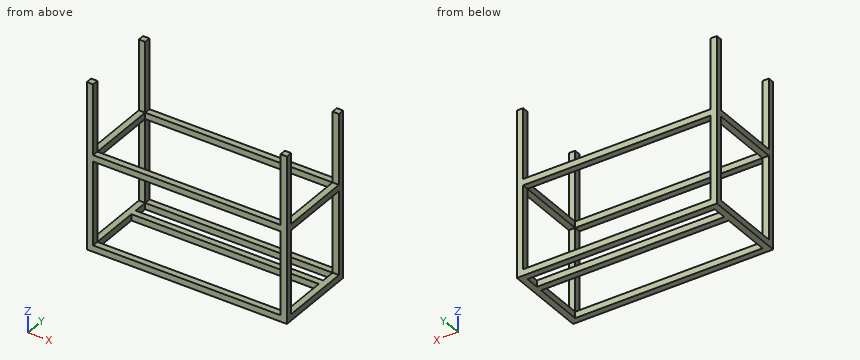
```python
from build123d import *

# Parameters (mm, degrees)
CROQUIS1_W              = 1200
CROQUIS1_H              = 500
CROQUIS1_W_2            = 1123.8
CROQUIS1_H_2            = 423.8
SALIENTE_EXTRUIR1_DEPTH = 38.1
CROQUIS2_W              = 38.1
CROQUIS2_H              = 38.1
SALIENTE_EXTRUIR2_DEPTH = 960
CROQUIS3_W              = 1123.8
CROQUIS3_H              = 38.1
SALIENTE_EXTRUIR4_DEPTH = 38.1
CROQUIS4_W              = 1123.8
CROQUIS4_H              = 38.1
SALIENTE_EXTRUIR5_DEPTH = 38.1
CROQUIS5_W              = 1123.8
CROQUIS5_H              = 38.1
SALIENTE_EXTRUIR6_DEPTH = 38.1
CROQUIS6_W              = 38.1
CROQUIS6_H              = 423.8
SALIENTE_EXTRUIR7_DEPTH = 38.1
CROQUIS7_W              = 38.1
CROQUIS7_H              = 423.8
SALIENTE_EXTRUIR8_DEPTH = 38.1


with BuildPart() as part:
    # Croquis1 → Saliente-Extruir1 (new body)
    with BuildSketch(Plane.XY):
        Rectangle(CROQUIS1_W, CROQUIS1_H)
        Rectangle(CROQUIS1_W_2, CROQUIS1_H_2, mode=Mode.SUBTRACT)
    extrude(amount=SALIENTE_EXTRUIR1_DEPTH)

    # Croquis2 → Saliente-Extruir2 (add)
    with BuildSketch(Plane.XY.offset(38.1)):
        with Locations((-580.95, 230.95)):
            Rectangle(CROQUIS2_W, CROQUIS2_H)
        with Locations((-580.95, -230.95)):
            Rectangle(CROQUIS2_W, CROQUIS2_H)
        with Locations((580.95, 230.95)):
            Rectangle(CROQUIS2_W, CROQUIS2_H)
        with Locations((580.95, -230.95)):
            Rectangle(CROQUIS2_W, CROQUIS2_H)
    extrude(amount=SALIENTE_EXTRUIR2_DEPTH)

    # Croquis3 → Saliente-Extruir4 (add)
    with BuildSketch(Plane(origin=(0, 0, 0), x_dir=(-1, 0, 0), z_dir=(0, 0, -1))):
        with Locations((0, 109.05)):
            Rectangle(CROQUIS3_W, CROQUIS3_H)
    extrude(amount=-SALIENTE_EXTRUIR4_DEPTH)

    # Croquis4 → Saliente-Extruir5 (add)
    with BuildSketch(Plane.XZ.offset(250)):
        with Locations((0, 557.15)):
            Rectangle(CROQUIS4_W, CROQUIS4_H)
    extrude(amount=-SALIENTE_EXTRUIR5_DEPTH)

    # Croquis5 → Saliente-Extruir6 (add)
    with BuildSketch(Plane(origin=(0, 250, 0), x_dir=(1, 0, 0), z_dir=(0, 1, 0))):
        with Locations((0, -557.15)):
            Rectangle(CROQUIS5_W, CROQUIS5_H)
    extrude(amount=-SALIENTE_EXTRUIR6_DEPTH)

    # Croquis6 → Saliente-Extruir7 (add)
    with BuildSketch(Plane.ZY.offset(600)):
        with Locations((557.15, 0)):
            Rectangle(CROQUIS6_W, CROQUIS6_H)
    extrude(amount=-SALIENTE_EXTRUIR7_DEPTH)

    # Croquis7 → Saliente-Extruir8 (add)
    with BuildSketch(Plane(origin=(600, 0, 0), x_dir=(0, 0, -1), z_dir=(1, 0, 0))):
        with Locations((-557.15, 0)):
            Rectangle(CROQUIS7_W, CROQUIS7_H)
    extrude(amount=-SALIENTE_EXTRUIR8_DEPTH)


solid = part.part
```
Build history of the part. All positions in model axes, mm. Give positions to 0.01 mm unless a question says otherwise; leave off trailing zeros. Loops run counter-clockwise (first coordinate to the right, second up) from the corner with the lowest first, then second, coordinate; pieces in that order, holes last. Notation, with made-up numbers: (-6, 59.25) - (1, 59.25) arc R15 cw to (1, 66.25) - close; hole circle Ø4 at (-11.75, 67.25). An arc over 180 degrees is marked (long way). Use a Markdown table: item, result.
(1) Band-saw the part on A-A (x = 41). Give the cut face in (y, z).
Taken from the geometry:
| item | result |
|---|---|
| outline | (-250, 0) - (-211.9, 0) - (-211.9, 38.1) - (-250, 38.1) - close; (-250, 538.1) - (-211.9, 538.1) - (-211.9, 576.2) - (-250, 576.2) - close; (90, 0) - (128.1, 0) - (128.1, 38.1) - (90, 38.1) - close; (211.9, 0) - (250, 0) - (250, 38.1) - (211.9, 38.1) - close; (211.9, 538.1) - (250, 538.1) - (250, 576.2) - (211.9, 576.2) - close |
(2) Band-saw the part on B-B (z = 887.5). Give the cut face in (x, y).
Taken from the geometry:
| item | result |
|---|---|
| outline | (-600, -250) - (-561.9, -250) - (-561.9, -211.9) - (-600, -211.9) - close; (-600, 211.9) - (-561.9, 211.9) - (-561.9, 250) - (-600, 250) - close; (561.9, -250) - (600, -250) - (600, -211.9) - (561.9, -211.9) - close; (561.9, 211.9) - (600, 211.9) - (600, 250) - (561.9, 250) - close |
(3) Wall check: line 1 along Z through (x, y) = (184.5, 217). Give the ranges that are in metal, low to high.
Taken from the geometry:
| item | result |
|---|---|
| line 1 | 0 to 38.1, 538.1 to 576.2 |
(4) Band-saw the part on C-C (y = 105). Give the cut face in (x, z), and give its area (3 significant figures).
Taken from the geometry:
| item | result |
|---|---|
| outline | (-600, 0) - (600, 0) - (600, 38.1) - (-600, 38.1) - close; (-600, 538.1) - (-561.9, 538.1) - (-561.9, 576.2) - (-600, 576.2) - close; (561.9, 538.1) - (600, 538.1) - (600, 576.2) - (561.9, 576.2) - close |
| area | 48,600 mm2 |
(5) Drop a flat-ended pin along its axis: pin 1 Ø11.5 at (x, y) = (67, -238) entering from +Z. Give the stop position or say it passes through.
Taken from the geometry:
| item | result |
|---|---|
| pin 1 | z = 576.2 |
(6) Band-saw the part on D-D (y = -136.5). Give the cut face in (x, z), and give its area (3 significant figures).
Taken from the geometry:
| item | result |
|---|---|
| outline | (-600, 0) - (-561.9, 0) - (-561.9, 38.1) - (-600, 38.1) - close; (-600, 538.1) - (-561.9, 538.1) - (-561.9, 576.2) - (-600, 576.2) - close; (561.9, 0) - (600, 0) - (600, 38.1) - (561.9, 38.1) - close; (561.9, 538.1) - (600, 538.1) - (600, 576.2) - (561.9, 576.2) - close |
| area | 5,810 mm2 |
